Autodesk Inventor part; units mm, degrees
ref_plane "YZ Plane" through (0, 0, 0) normal (1, 0, 0) x (0, 1, 0)
ref_plane "XZ Plane" through (0, 0, 0) normal (0, 1, 0) x (-1, 0, 0)
ref_plane "XY Plane" through (0, 0, 0) normal (0, 0, 1) x (1, 0, 0)
sketch "Sketch1" plane through (0, 0, 0) normal (1, 0, 0) x (0, 1, 0)
  line L0 (0, 0) -> (12, 0)
  line L1 (12, 0) -> (12, 12)
  line L2 (12, 12) -> (0, 12)
  line L3 (0, 12) -> (0, 0)
  line L4 (-1.5, 13.5) -> (13.5, 13.5)
  line L5 (13.5, 13.5) -> (13.5, -1.5)
  line L6 (13.5, -1.5) -> (-1.5, -1.5)
  line L7 (-1.5, -1.5) -> (-1.5, 13.5)
  dimension "d0" = 1.5
  dimension "d1" = 12
  dimension "d2" = 12
extrude "Extrusion1" add sketch "Sketch1" along normal blind 30 and the other way blind 15
sketch "Sketch2" plane through (0, -1.5, 13.5) normal (0, 0, 1) x (1, 0, 0)
  line L0 (0, 0) -> (0, 15)
  line L1 (0, 0) -> (30, 0)
  circle A0 centre (-16, 7.5) radius 16
  circle A1 centre (-16, 7.5) radius 30
  circle A2 centre (14, 7.5) radius 2
  point P0 (0, 1.5)
  dimension "d17" = 60
  dimension "d8" = 32
  dimension "d9" = 16
  dimension "d18" = 4
sketch "Sketch4" plane through (0, 0, 0) normal (-1, 0, 0) x (0, 0, 1)
  line L0 (0, 0) -> (12, 0)
  line L1 (12, 0) -> (12, 12)
  line L2 (12, 12) -> (0, 12)
  line L3 (0, 12) -> (0, 0)
  line L4 (-1.5, -1.5) -> (13.5, -1.5)
  line L5 (13.5, -1.5) -> (13.5, 13.5)
  line L6 (13.5, 13.5) -> (-1.5, 13.5)
  line L7 (-1.5, 13.5) -> (-1.5, -1.5)
extrude "Extrusion2" add sketch "Sketch4" along normal blind 10
extrude "Extrusion3" cut sketch "Sketch2" against normal through all contours A0
extrude "Extrusion4" cut sketch "Sketch2" along normal through all both and the other way through all contours A2 A1 | A1 A2 picked at (14.5954, 6.9828) picked at (13.3724, 7.0462)
equation "\"d0\" = ZártSzelvényFalVastagság"
equation "\"d1\" = ZártSzelvényBelsőÁtmérő"
equation "\"d2\" = ZártSzelvényBelsőÁtmérő"
equation "\"d17\" = 2 * PorvedoRogzitesJatekSugara"
equation "\"d8\" = CsapágyHázKülsőÁtmérő"
equation "\"d9\" = 0.5 * CsapágyHázKülsőÁtmérő"
equation "\"ZártSzelvényFalVastagság\" = 1.5"
equation "\"ZártSzelvényBelsőÁtmérő\" = 12"
equation "\"CsapágyHázKülsőÁtmérő\" = 32"
equation "\"ZártSzelvényKülsőÁtmérő\" = 15"
equation "\"CsapágyBelsőÁtmérő\" = 12"
equation "\"CsapágyKülsőÁtmérő\" = 28"
equation "\"CsapágyHázBelsőÁtmérő\" = 26"
equation "\"CsapágyHázHoszza\" = 45"
equation "\"CsapágySzélesége\" = 8"
properties part number "KétvégenMartSzelvény" material "Acetal Resin, Black"
Read the model definition and answer for the solid it produces. Units are mm, in the model's axes. A direction names the side the tool comes from. Coordinates: 2 decimals unless noted, no trailing zeros. Write each loop counter-clockwise with the first axis right and the second up, starting at its lowest first coordinate (ties: lowest second). Pieces come first, ordered by that corner, then holes. Notation, with made-up numbers: (-29, 17.5) - (10, 17.5) arc R23 ccw to (10, 36.5) - close; hole circle Ø2 at (41, 45). An arc over 180 degrees is marked (long way). Answer as a JSON object with one key per item and string values. Group by question number.
1. A cutting plane is placed at C-C (y = 6). Determine the outline of the cut face in (x, z).
2. The mould has two halves that part along Y. Classify faces 3 (the flat face through (30, -1, 6)), 4 (the flat face through (14, -1.5, 6)), 5 (the flat face through (14, 9, 12)): +Y half, -Y half, draft (parallel to the pull), parting line (faces both ways), or undercut.
3. Which of the six approach directions +Z, -Z, +X, -X, +Y, -Y give full straight-line access (tool end or side, diameter ignored) to faces 1 (the flat face through (14, 12, 6)), 2 (the flat face through (17, 6, -1.5))?
4. A cutting plane is placed at B-B (z = 8.75). Determine the outline of the cut face in (x, y).
5. A cutting plane is placed at D-D (y = 9.75). Determine the outline of the cut face in (x, z), plus the area to 3 significant figures.
6. Consider L1, parallel to Z at x = 6, y = 5.75; L2, parallel to Y at x = 14, z = 12.8. Determine where each line is inside the solid, lowest interval first. Write a range as [from, to].
7. A cutting plane is placed at A-A (x = 14). Determine the outline of the cut face in (y, z), plus the area to 3 significant figures.
8. Each of these flat-tipped pins is pushed along its axis until it touches: P1, Ø8, axis at y = 3.5, z = 1, coming from the -X side; P2, Ø6, axis at y = 5.5, z = 4, coming from the -X side. Where does it stop, or does it pass through?
Worked out:
{
 "1": {"outline": "(0, -1.5) - (12, -1.5) - (12, 0) - (0, 0) - close; (0, 12) - (12, 12) - (12, 13.5) - (0, 13.5) - close; (16, -1.5) - (30, -1.5) - (30, 0) - (16, 0) - close; (16, 12) - (30, 12) - (30, 13.5) - (16, 13.5) - close"},
 "2": {"face 3": "draft", "face 4": "-Y half", "face 5": "undercut"},
 "3": {"face 1": "+X, -X", "face 2": "-Z, +X, -X, +Y, -Y"},
 "4": {"outline": "(-1.87, -1.5) - (30, -1.5) - (30, 0) - (-1.17, 0) arc R16 cw to start; (-1.87, 13.5) arc R16 cw to (-1.17, 12) - (30, 12) - (30, 13.5) - close"},
 "5": {"outline": "(-0.45, -1.5) - (30, -1.5) - (30, 0) - (-0.45, 0) - close; (-0.45, 12) - (30, 12) - (30, 13.5) - (-0.45, 13.5) - close", "area": "91.3 mm²"},
 "6": {"L1": "z = [-1.5, 0], [12, 13.5]", "L2": "y = [-1.5, 4], [8, 13.5]"},
 "7": {"outline": "(-1.5, -1.5) - (4, -1.5) - (4, 0) - (0, 0) - (0, 12) - (4, 12) - (4, 13.5) - (-1.5, 13.5) - close; (8, -1.5) - (13.5, -1.5) - (13.5, 13.5) - (8, 13.5) - (8, 12) - (12, 12) - (12, 0) - (8, 0) - close", "area": "69.0 mm²"},
 "8": {"P1": "stops at x = -1.38", "P2": "passes through"}
}
